Work out the finished part from the listing and answer in its coordinate system (mm). A direction names the side the tool comes from. Coordinates: 2 decimals unless noted, no trailing zeros. Order: outer loops, then holes, each group sorted by start corner. A loop starts at its lowest first (then second) coordinate and runs counter-clockwise, first axis right, second up. Notation, with made-up numbers: M 24.25,-40 L 59.25,-40 A23 ccw 59.25,-15 Z; hole C 60.25,56.25 d5. An arc over 180 degrees is marked long. Use a Markdown table: item, result. Add a question column.
from build123d import *

# Parameters (mm, degrees)
SKETCH_1_W                       = 160
SKETCH_1_H                       = 70
SM_BASE_FLANGE_1_DEPTH           = 10
SM_EDGE_FLANGE_1_STRIP_W         = 41.4732
SM_EDGE_FLANGE_1_STRIP_H         = 10
SM_EDGE_FLANGE_1_STRIP_CUT_DEPTH = 70
SM_EDGE_FLANGE_1_DEPTH           = 70
EXTRUDE_1_DEPTH                  = 5
FILLET_1_R                       = 10
CUT_EXTRUDE_1_DEPTH              = 10
FILLET_2_R                       = 5
SKETCH_11_R                      = 3.3
CUT_EXTRUDE_2_DEPTH              = 10
SKETCH_12_R                      = 3.3
CUT_EXTRUDE_3_DEPTH              = 10
SKETCH_13_R                      = 10
SKETCH_13_R_2                    = 10.151646836
CUT_EXTRUDE_4_DEPTH              = 10


# Sheet-metal steps are written as plain solids
with BuildPart() as part:
    # Sketch 1 → 基体-法兰1 (new body)
    with BuildSketch(Plane.XY):
        Rectangle(SKETCH_1_W, SKETCH_1_H)
    extrude(amount=-SM_BASE_FLANGE_1_DEPTH)

    # 边线-法兰1 strip (across the edge) → 边线-法兰1 strip cut (cut)
    with BuildSketch(Plane(origin=(-80, 35, 0), x_dir=(1, 0, 0), z_dir=(0, -1, 0))):
        with Locations((-10, -5)):
            Rectangle(SM_EDGE_FLANGE_1_STRIP_W, SM_EDGE_FLANGE_1_STRIP_H)
    extrude(amount=SM_EDGE_FLANGE_1_STRIP_CUT_DEPTH, mode=Mode.SUBTRACT)

    # 边线-法兰1 section (across the edge) → 边线-法兰1 (add)
    with BuildSketch(Plane(origin=(-80, 35, 0), x_dir=(1, 0, 0), z_dir=(0, -1, 0))):
        with BuildLine():
            Line((0, 0.7366), (0, 150))
            Line((0, 150), (10, 150))
            Line((10, 150), (10, 0.7366))
            ThreePointArc((10, 0.7366), (10.215745145, 0.215745145), (10.7366, 0))
            Line((10.7366, 0), (10.7366, -10))
            ThreePointArc((10.7366, -10), (3.144677333, -6.855322667), (0, 0.7366))
        make_face()
    extrude(amount=SM_EDGE_FLANGE_1_DEPTH)

    # 草图9 → 凸台-拉伸1 (add, symmetric)
    with BuildSketch(Plane(origin=(0, 0, 0), x_dir=(1, 0, 0), z_dir=(0, 1, 0))):
        with BuildLine():
            Line((-70, -150), (-54, -150))
            Line((-54, -150), (80, -16))
            Line((80, -16), (80, 0))
            Line((80, 0), (-69.2634, 0))
            ThreePointArc((-69.2634, 0), (-69.784254855, -0.215745145), (-70, -0.7366))
            Line((-70, -0.7366), (-70, -150))
        make_face()
    extrude(amount=EXTRUDE_1_DEPTH, both=True)

    # 圆角1
    fillet_1_edges = [part.edges().sort_by_distance(p)[0] for p in [
        (-75, 35, 150),
        (-75, -35, 150),
        (-54, 0, 150),
        (80, 0, 16),
        (80, -35, -5),
        (80, 35, -5),
    ]]
    fillet(fillet_1_edges, radius=FILLET_1_R)

    # 草图10 → 切除-拉伸1 (cut)
    with BuildSketch(Plane(origin=(0, 5, 0), x_dir=(1, 0, 0), z_dir=(0, 1, 0))):
        Polygon((-42, -98.402020254), (28.402020254, -28), (-42, -28), align=None)
    extrude(amount=-CUT_EXTRUDE_1_DEPTH, mode=Mode.SUBTRACT)

    # 圆角2
    fillet_2_edges = [part.edges().sort_by_distance(p)[0] for p in [
        (-42, 0, 98.402020254),
        (-42, 0, 28),
        (28.402020254, 0, 28),
    ]]
    fillet(fillet_2_edges, radius=FILLET_2_R)

    # 草图11 → 切除-拉伸2 (cut)
    with BuildSketch(Plane(origin=(-70, 0, 0), x_dir=(0, 0, -1), z_dir=(1, 0, 0))):
        with Locations((-50, 20)):
            Circle(SKETCH_11_R)
        with Locations((-10, 20)):
            Circle(SKETCH_11_R)
        with Locations((-10, -20)):
            Circle(SKETCH_11_R)
        with Locations((-50, -20)):
            Circle(SKETCH_11_R)
        with BuildLine():
            Line((-134, 23.3), (-126, 23.3))
            ThreePointArc((-126, 23.3), (-122.7, 20), (-126, 16.7))
            Line((-126, 16.7), (-134, 16.7))
            ThreePointArc((-134, 16.7), (-137.3, 20), (-134, 23.3))
        make_face()
        with BuildLine():
            Line((-86, 16.7), (-94, 16.7))
            ThreePointArc((-94, 16.7), (-97.3, 20), (-94, 23.3))
            Line((-94, 23.3), (-86, 23.3))
            ThreePointArc((-86, 23.3), (-82.7, 20), (-86, 16.7))
        make_face()
        with BuildLine():
            Line((-86, -23.3), (-94, -23.3))
            ThreePointArc((-94, -23.3), (-97.3, -20), (-94, -16.7))
            Line((-94, -16.7), (-86, -16.7))
            ThreePointArc((-86, -16.7), (-82.7, -20), (-86, -23.3))
        make_face()
        with BuildLine():
            Line((-126, -23.3), (-134, -23.3))
            ThreePointArc((-134, -23.3), (-137.3, -20), (-134, -16.7))
            Line((-134, -16.7), (-126, -16.7))
            ThreePointArc((-126, -16.7), (-122.7, -20), (-126, -23.3))
        make_face()
    extrude(amount=-CUT_EXTRUDE_2_DEPTH, mode=Mode.SUBTRACT)

    # 草图12 → 切除-拉伸3 (cut)
    with BuildSketch(Plane.XY):
        with Locations((-40, -20)):
            Circle(SKETCH_12_R)
        with Locations((-40, 20)):
            Circle(SKETCH_12_R)
        with Locations((40, 20)):
            Circle(SKETCH_12_R)
        with Locations((40, -20)):
            Circle(SKETCH_12_R)
        with Locations((0, -20)):
            Circle(SKETCH_12_R)
        with Locations((0, 20)):
            Circle(SKETCH_12_R)
    extrude(amount=-CUT_EXTRUDE_3_DEPTH, mode=Mode.SUBTRACT)

    # 草图13 → 切除-拉伸4 (cut)
    with BuildSketch(Plane(origin=(0, 5, 0), x_dir=(1, 0, 0), z_dir=(0, 1, 0))):
        with Locations(Location((3.100505063, -73.100505063, 0), (0, 0, 270))):
            Circle(SKETCH_13_R)
        with Locations(Location((-55, -128, 0), (0, 0, 270))):
            Circle(SKETCH_13_R_2)
    extrude(amount=-CUT_EXTRUDE_4_DEPTH, mode=Mode.SUBTRACT)


solid = part.part
(1) Which of the six approach directions +Z, -Z, +X, -X, +Y, -Y give full straight-line access (tool end or side, diameter ignored) to faces 4 (the flat face through (4, -20, 0)), 5 (the flat face through (-32, -35, -1)), 6 (the cylindrical face through (-74.9, 20.1, 82.7)), 7 (the flat face through (-42, 0, 59))?
(2) Straight lines are drawn through the part: line 1 (Y direction, x = 0, z = -2.25); line 2 (X direction, y = -29, z = 119); line 3 (Z direction, x = -65.5, y = 31). For each, find the intervals that lie inside material, in ascending order.
(3) The mould has two halves that part along X. Classify faces 1 (the cylindrical face through (-74.9, -19.9, 53.3)), 2 (the cylindrical face through (3.54, 0.07, 63.11)), 3 (the cylindrical face through (-54.37, 0.07, 149.26)): pulls with the +X half, pulls with the -X half, needs draft (parallel to the pull), parting line crosses it, or undercut.
(4) A cutting plane is placed at C-C on z = 24.5. Write down the section's boundary in (x, y), plus the area to 4 significant figures.
(5) A cutting plane is placed at D-D on x = -55. Write down the section's boundary in (y, z).
(6) Given P1, Ø1.5, axis at x = 8.5, z = 46, coming from the -Y side; P2, Ø24, axis at x = 6.5, y = -15.5, coming from the +Z side; P3, Ø8, axis at y = 13, z = 66, coming from the +X side; P4, Ø3, axis at x = -19.5, z = 28, coming from the -Y side, each flat-ended and moving along its own axis, determine where each tip first touches the part or whether it passes through.
(7) A cutting plane is placed at B-B on y = -12. Write down the section's boundary in (x, z).
(8) A cutting plane is placed at A-A on x = 40. Write down the section's boundary in (y, z).
From the geometry:
| question | item | result |
|---|---|---|
| 1 | face 4 | +Z, +X, -Y |
| 1 | face 5 | +Z, -Z, +X, -X, -Y |
| 1 | face 6 | +X, -X |
| 1 | face 7 | +Y, -Y |
| 2 | line 1 | y = -35 to -23.3, -16.7 to 16.7, 23.3 to 35 |
| 2 | line 2 | x = -80 to -70 |
| 2 | line 3 | z = -10 to 0 |
| 3 | face 1 | needs draft |
| 3 | face 2 | undercut |
| 3 | face 3 | pulls with the +X half |
| 4 | outline | M -80,-35 L -70,-35 L -70,-5 L 71.5,-5 L 71.5,5 L -70,5 L -70,35 L -80,35 Z |
| 4 | area | 2,115 mm2 |
| 5 | outline | M -35,-10 L 35,-10 L 35,0 L 5,0 L 5,117.85 L -5,117.85 L -5,0 L -35,0 Z; M -5,138.15 L 5,138.15 L 5,149.49 L -5,149.49 Z |
| 6 | P1 | passes through |
| 6 | P2 | stops at z = 95.31 |
| 6 | P3 | stops at x = -70 |
| 6 | P4 | stops at y = -5 |
| 7 | outline | M -80,0.74 A10.74 ccw -69.26,-10 L 80,-10 L 80,0 L -69.26,0 A0.74 cw -70,0.74 L -70,150 L -80,150 Z |
| 8 | outline | M -35,-10 L -23.3,-10 L -23.3,0 L -35,0 Z; M -16.7,-10 L 16.7,-10 L 16.7,0 L 5,0 L 5,56 L -5,56 L -5,0 L -16.7,0 Z; M 23.3,-10 L 35,-10 L 35,0 L 23.3,0 Z |
